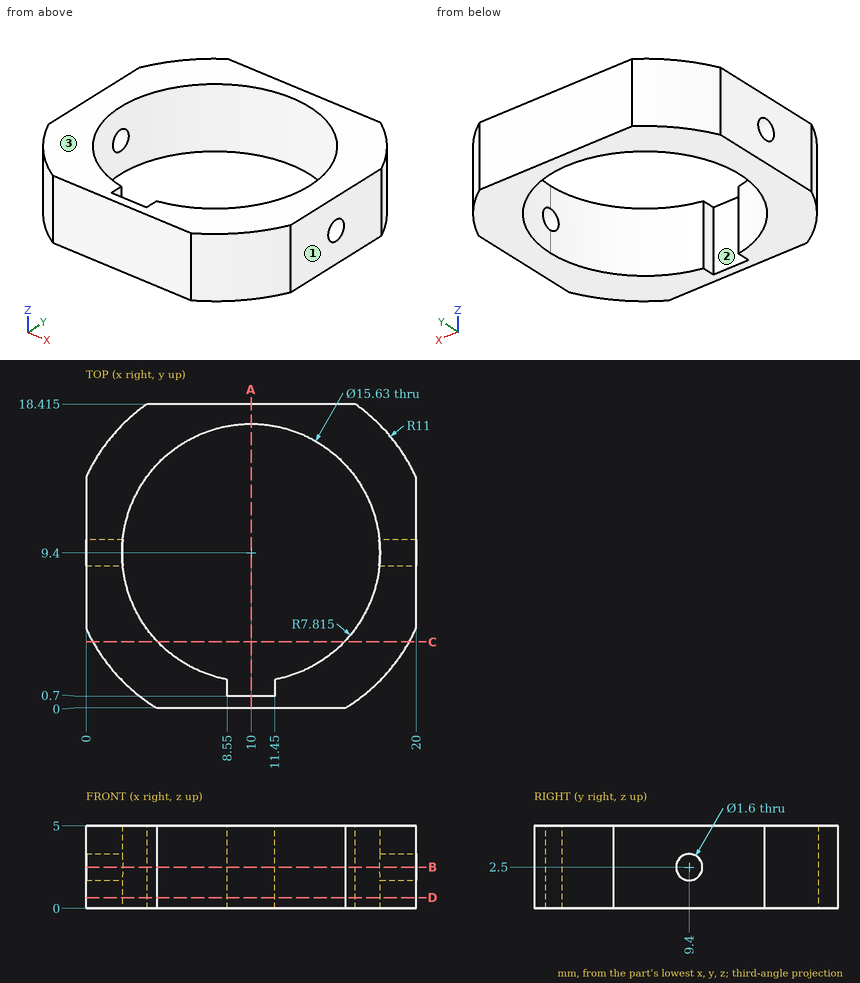
Drawing for the job (mm, zero at the part's lowest x, y, z). Round coordinates to 2 decimals unless told otherwise and drop trailing zeros. Order: outer loops, then holes, each group sorted by start corner. A loop starts at its lowest first (then second) coordinate and runs counter-clockwise, first axis right, second up. Notation, with made-up numbers: M 51,-24.75 L 71,-24.75 A19 ccw 71,-11.75 Z; hole C -31.5,40.5 d2. An arc over 180 degrees is marked long. Use one line per item in the form item = value.
Q1. Two-plate mould, pull along X, no slides. Class the marked faces 1, 2 and 3: +X half, -X half, draft (parallel to the pull), parting line (faces both ways), or undercut.
Recorded:
face_1 = +X half
face_2 = undercut
face_3 = draft
Q2. Probe L1, parallel to Y at x = 10, z = 1.65 (3 decimals); L2, parallel to Z at x = 1.4, y = 9.4; L3, parallel to X at y = 9.25, z = 3.4. List the from-to ranges inside material, lowest first.
Recorded:
L1 = 0 to 0.7, 17.215 to 18.415
L2 = 0 to 1.7, 3.3 to 5
L3 = 0 to 2.19, 17.81 to 20
Q3. Saw through at B-B on z = 2.5. Give the cut face in (x, y) (3 decimals), then the cut area to 3 significant figures.
Recorded:
outline = M 0,4.817 A11 ccw 4.287,0 L 15.713,0 A11 ccw 20,4.817 L 20,8.6 L 17.774,8.6 A7.815 cw 11.45,1.721 L 11.45,0.7 L 8.55,0.7 L 8.55,1.721 A7.815 cw 2.226,8.6 L 0,8.6 Z; M 0,10.2 L 2.226,10.2 A7.815 cw 17.774,10.2 L 20,10.2 L 20,13.983 A11 ccw 16.303,18.415 L 3.697,18.415 A11 ccw 0,13.983 Z
area = 137 mm^2
Q4. Flat gauge pins, fed straight in: P1, Ø1.5, axis at y = 2, z = 1, coming from the +X side; P2, Ø5, axis at x = 10.5, y = 4, coming from the -Z side; P3, Ø1.1, axis at y = 1.5, z = 2, coming from the -X side; P4, Ø0.5, axis at y = 1.5, z = 1.5, coming from the +X side. Where does each tip first touch, or does it go through?
Recorded:
P1 = 18.76
P2 = 0
P3 = 1.82
P4 = 17.9
Q5. Saw through at A-A on x = 10. Give the cut face in (y, z) (3 decimals), then the cut area to 3 significant figures.
Recorded:
outline = M 0,0 L 0.7,0 L 0.7,5 L 0,5 Z; M 17.215,0 L 18.415,0 L 18.415,5 L 17.215,5 Z
area = 9.50 mm^2
Q6. Saw through at D-D on z = 0.65. Give the cut face in (x, y) (3 decimals), then the cut area to 3 significant figures.
Recorded:
outline = M 0,4.817 A11 ccw 4.287,0 L 15.713,0 A11 ccw 20,4.817 L 20,13.983 A11 ccw 16.303,18.415 L 3.697,18.415 A11 ccw 0,13.983 Z; hole M 8.55,0.7 L 11.45,0.7 L 11.45,1.721 A7.815 ccw long 8.55,1.721 Z
area = 144 mm^2
Q7. Saw through at C-C on y = 4. Give the cut face in (x, z), then the cut area to 3 significant figures.
Recorded:
outline = M 0.42,0 L 4.35,0 L 4.35,5 L 0.42,5 Z; M 15.65,0 L 19.58,0 L 19.58,5 L 15.65,5 Z
area = 39.3 mm^2
